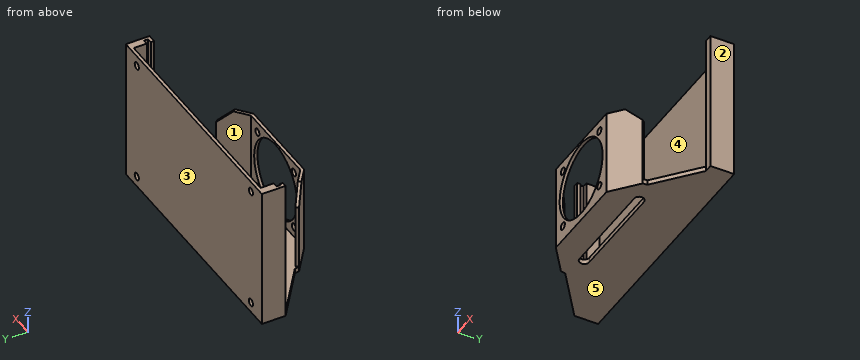
```python
from build123d import *

# Parameters (mm, degrees)
BOSS_EXTRUDE1_DEPTH = 85
BOSS_EXTRUDE2_DEPTH = 3
EXTRUDE_THIN1_DEPTH = 53
CHAMFER1_SIZE       = 10
CHAMFER2_SIZE       = 2
CUT_EXTRUDE1_DEPTH  = 53
SKETCH6_R           = 23.5
SKETCH6_R_2         = 2.25
CUT_EXTRUDE2_DEPTH  = 53
SKETCH7_R           = 2.25
CUT_EXTRUDE3_DEPTH  = 53


with BuildPart() as part:
    # Sketch1 → Boss-Extrude1 (new body)
    with BuildSketch(Plane.XY):
        Polygon((0, 0), (69.5, 0), (69.5, -8), (72.5, -8), (72.5, -10.5), (69.5, -10.5), (69.5, -12.5), (74.5, -12.5), (74.5, -6), (74.5, 2), (71.5, 2), (0, 2), (-71.5, 2), (-74.5, 2), (-74.5, -6), (-74.5, -12.5), (-71.5, -12.5), (-71.5, -10.5), (-72.5, -10.5), (-72.5, -8), (-69.5, -8), (-69.5, 0), align=None)
    extrude(amount=BOSS_EXTRUDE1_DEPTH)

    # Sketch2 → Boss-Extrude2 (add)
    with BuildSketch(Plane(origin=(0, 0, 0), x_dir=(-1, 0, 0), z_dir=(0, 0, -1))):
        Polygon((-27, -48), (27, -48), (74.5, -12.5), (74.5, 2), (-74.5, 2), (-74.5, -12.5), (-69.5, -12.5), align=None)
    extrude(amount=BOSS_EXTRUDE2_DEPTH)

    # Sketch4 → Extrude-Thin1 (add)
    with BuildSketch(Plane(origin=(0, 0, -3), x_dir=(-1, 0, 0), z_dir=(0, 0, -1))):
        Polygon((43.020213309, -36.026998474), (27, -48), (-27, -48), (-42.349613383, -35.178558233), (-43.63175756, -36.713519571), (-27.725407751, -50), (27.664793483, -50), (44.217513462, -37.629019805), align=None)
    extrude(amount=-EXTRUDE_THIN1_DEPTH)

    # Chamfer1
    chamfer1_edges = [part.edges().sort_by_distance(p)[0] for p in [
        (-43.618863385, -36.82800914, 50),
        (42.990685472, -35.946038902, 50),
    ]]
    chamfer(chamfer1_edges, length=CHAMFER1_SIZE)

    # Chamfer2
    chamfer2_edges = [part.edges().sort_by_distance(p)[0] for p in [
        (-43.020213309, -36.026998474, -1.5),
        (42.349613383, -35.178558233, -1.5),
    ]]
    chamfer(chamfer2_edges, length=CHAMFER2_SIZE - 0.0001)  # a hair under: the kernel refuses the full size

    # Sketch5 → Cut-Extrude1 (cut)
    with BuildSketch(Plane.XY):
        with BuildLine():
            Line((-30, -28.267007474), (30, -28.267007474))
            ThreePointArc((30, -28.267007474), (33, -31.267007474), (30, -34.267007474))
            Line((30, -34.267007474), (-30, -34.267007474))
            ThreePointArc((-30, -34.267007474), (-33, -31.267007474), (-30, -28.267007474))
        make_face()
    extrude(amount=-CUT_EXTRUDE1_DEPTH, mode=Mode.SUBTRACT)

    # Sketch6 → Cut-Extrude2 (cut)
    with BuildSketch(Plane(origin=(0, -48, 0), x_dir=(1, 0, 0), z_dir=(0, 1, 0))):
        with Locations(Location((0, -25, 0), (0, 0, 270))):
            Circle(SKETCH6_R)
        with Locations(Location((20, -43.518518519, 0), (0, 0, 270))):
            Circle(SKETCH6_R_2)
        with Locations(Location((-20, -43.518518519, 0), (0, 0, 270))):
            Circle(SKETCH6_R_2)
        with Locations(Location((-20, -6.481481481, 0), (0, 0, 270))):
            Circle(SKETCH6_R_2)
        with Locations(Location((20, -6.481481481, 0), (0, 0, 270))):
            Circle(SKETCH6_R_2)
    extrude(amount=-CUT_EXTRUDE2_DEPTH, mode=Mode.SUBTRACT)

    # Sketch7 → Cut-Extrude3 (cut)
    with BuildSketch(Plane(origin=(0, 2, 0), x_dir=(1, 0, 0), z_dir=(0, 1, 0))):
        with Locations(Location((62.5, -78.5, 0), (0, 0, 270))):
            Circle(SKETCH7_R)
        with Locations(Location((62.5, -3.5, 0), (0, 0, 270))):
            Circle(SKETCH7_R)
        with Locations(Location((-62.5, -3.5, 0), (0, 0, 270))):
            Circle(SKETCH7_R)
        with Locations(Location((-62.5, -78.5, 0), (0, 0, 270))):
            Circle(SKETCH7_R)
    extrude(amount=-CUT_EXTRUDE3_DEPTH, mode=Mode.SUBTRACT)


solid = part.part
```
Model file for the job. Use its own axes, mm. Face numbers are marked on the shaded views. A direction names the side the tool comes from. Give positions to 0.01 mm unless a question says otherwise; leave off trailing zeros. Write each loop counter-clockwise with the first axis right and the second up, starting at its lowest first coordinate (ties: lowest second). Pieces come first, ordered by that corner, then holes. Notation, with made-up numbers: M -13.75,-24.5 L 12.25,-24.5 A28 cw 12.25,5.5 Z; hole C -0.75,88.25 d10. An arc over 180 degrees is marked long. Use a Markdown table: item, result.
1) Cut at A-A (z = 78.5). List the corners of the cut face in (x, y), and give its area (3 significant figures).
Responses:
| item | result |
|---|---|
| outline | M -74.5,-12.5 L -71.5,-12.5 L -71.5,-10.5 L -72.5,-10.5 L -72.5,-8 L -69.5,-8 L -69.5,0 L -64.75,0 L -64.75,2 L -74.5,2 Z; M -60.25,0 L 60.25,0 L 60.25,2 L -60.25,2 Z; M 64.75,0 L 69.5,0 L 69.5,-8 L 72.5,-8 L 72.5,-10.5 L 69.5,-10.5 L 69.5,-12.5 L 74.5,-12.5 L 74.5,2 L 64.75,2 Z |
| area | 386 mm2 |
2) Cut at B-B (x = -62.5). List the corners of the cut face in (y, z), and give its area (3 significant figures).
Responses:
| item | result |
|---|---|
| outline | M -21.47,-3 L 2,-3 L 2,1.25 L 0,1.25 L 0,0 L -21.47,0 Z; M 0,5.75 L 2,5.75 L 2,76.25 L 0,76.25 Z; M 0,80.75 L 2,80.75 L 2,85 L 0,85 Z |
| area | 222 mm2 |
3) Drill centre lines: line 1 (X direction, y = -6.5, z = 32); line 2 (X direction, y = -11, z = 71.5); line 3 (X direction, y = 1, z = 3). Where is each one in solid material? Low to high. Write a range as from..to.
Responses:
| item | result |
|---|---|
| line 1 | x = -74.5..-69.5, 69.5..74.5 |
| line 2 | x = -74.5..-71.5, 69.5..74.5 |
| line 3 | x = -74.5..-64.69, -60.31..60.31, 64.69..74.5 |
4) Cut at C-C (y = -5.5). List the corners of the cut face in (x, z).
Responses:
| item | result |
|---|---|
| outline | M -74.5,-3 L 74.5,-3 L 74.5,85 L 69.5,85 L 69.5,0 L -69.5,0 L -69.5,85 L -74.5,85 Z |
5) Cut at D-D (x = 20). List the corners of the cut face in (y, z).
Responses:
| item | result |
|---|---|
| outline | M -50,-3 L -34.27,-3 L -34.27,0 L -48,0 L -48,4.23 L -50,4.23 Z; M -50,8.73 L -48,8.73 L -48,12.66 L -50,12.66 Z; M -50,37.34 L -48,37.34 L -48,41.27 L -50,41.27 Z; M -50,45.77 L -48,45.77 L -48,50 L -50,50 Z; M -28.27,-3 L 2,-3 L 2,85 L 0,85 L 0,0 L -28.27,0 Z |
6) Pull direction Y, two halves, no side cores. Call the marked faces 1, 2 and 3: +Y half, -Y half, draft (parallel to the pull), parting line (faces both ways), or undercut.
Responses:
| item | result |
|---|---|
| face 1 | undercut |
| face 2 | draft |
| face 3 | +Y half |
7) Tool access for the marked faces 4 and 5: list every direction of +Z, -Z, +X, -X, +Y, -Y with a clear straight run to the whole face (end or side of a thin tool).
Responses:
| item | result |
|---|---|
| face 4 | +Z |
| face 5 | -Z, +X, -X, +Y, -Y |
8) Pin check, flat tips, straight feed: pin 1 (1 mm diameter, centred on y = -40, z = 17, fed in from -X); pin 2 (3.5 mm diameter, centred on x = 70.5, z = 23, fed in from -Y); pin 3 (2.5 mm diameter, centred on x = -62.5, z = 78.5, fed in from +Y); pin 4 (12 mm diameter, centred on y = -40, z = 55.5, fed in from -X). Stop position of each tip, or through.
Responses:
| item | result |
|---|---|
| pin 1 | stops at x = -41.71 |
| pin 2 | stops at y = -12.5 |
| pin 3 | passes through |
| pin 4 | stops at x = -35.3 |
